```python
from build123d import *

# Parameters (mm, degrees)
SKETCH_1_W                         = 7.5
SKETCH_1_H                         = 4.2
EXTRUDE_1_DEPTH                    = 6
CUT_EXTRUDE_1_DEPTH                = 5
CUT_EXTRUDE_2_DEPTH                = 11.482843126
EXTRUDE_6_DEPTH                    = 1.1
CUT_EXTRUDE_3_REACH                = 12.483
SKETCH_5_W                         = 5.3
SKETCH_5_H                         = 4.3
EXTRUDE_3_REACH                    = 12.131
EXTRUDE_5_REACH                    = 13.88
SKETCH_11_W                        = 2
SKETCH_11_H                        = 4.2
SKETCH_11_W_2                      = 0.8
SKETCH_11_H_2                      = 0.8
CUT_EXTRUDE_5_DEPTH                = 0.1
SKETCH_15_R                        = 0.05
CUT_EXTRUDE_6_DEPTH                = 0.1
CUT_EXTRUDE_7_DEPTH                = 0.2
SKETCH_7_W                         = 0.6
SKETCH_7_H                         = 0.6
EXTRUDE_4_DEPTH                    = 5.5
SKETCH_18_W                        = 0.6
SKETCH_18_H                        = 0.6
CHAMFER_6_SIZE                     = 0.2
PATTERN_LINEAR_1_COUNT             = 2
PATTERN_LINEAR_1_PITCH             = 2.5
CHAMFER_6_OF_PATTERN_LINEAR_1_SIZE = 0.2
CUT_EXTRUDE_4_REACH                = 12.131
SKETCH_20_W                        = 0.6
SKETCH_20_H                        = 0.3
CUT_EXTRUDE_9_DEPTH                = 0.9
CHAMFER_5_SIZE                     = 0.3
SKETCH_19_R                        = 0.05
CUT_EXTRUDE_8_DEPTH                = 3.2


with BuildPart() as part:
    # Эскиз1 → Бобышка-Вытянуть1 (new body)
    with BuildSketch(Plane(origin=(0, 0, 0), x_dir=(1, 0, 0), z_dir=(0, 1, 0))):
        with Locations((3.75, -2.1)):
            Rectangle(SKETCH_1_W, SKETCH_1_H)
    extrude(amount=EXTRUDE_1_DEPTH)

    # Эскиз2 → Вырез-Вытянуть1 (cut)
    with BuildSketch(Plane(origin=(0, 6, 0), x_dir=(1, 0, 0), z_dir=(0, 1, 0))):
        Polygon((0.5, -0.9), (7, -0.9), (7, -1.9), (6.4, -1.9), (6.4, -3.7), (1.1, -3.7), (1.1, -1.9), (0.5, -1.9), align=None)
    extrude(amount=-CUT_EXTRUDE_1_DEPTH, mode=Mode.SUBTRACT)

    # Эскиз3 → Вырез-Вытянуть2 (cut, through all)
    with BuildSketch(Plane.ZY):
        Polygon((2.2, 6), (2.2, 1.5), (2.7, 1.5), (3.1, 3.459591794), (3.1, 4.021282026), (2.8, 4.285857157), (2.8, 4.585857157), (3.5, 5.3), (4.2, 5.3), (4.2, 6), align=None)
    extrude(amount=-CUT_EXTRUDE_2_DEPTH, mode=Mode.SUBTRACT)

    # Эскиз16 → Бобышка-Вытянуть6 (add)
    with BuildSketch(Plane(origin=(7.5, 0, 0), x_dir=(0, 0, -1), z_dir=(1, 0, 0))):
        Polygon((-2.4, 0), (-1.3, -2.2), (0, -2.2), (0, 0), align=None)
    extrude_6 = extrude(amount=-EXTRUDE_6_DEPTH)

    # Зеркальное отражение2: Бобышка-Вытянуть6 across plane
    add(extrude_6.mirror(Plane(origin=(3.75, 0, 0), x_dir=(0, 0, 1), z_dir=(1, 0, 0))))

    # Эскиз5 → Вырез-Вытянуть3 (cut, up to next)
    with BuildSketch(Plane.XY.offset(4.2), mode=Mode.PRIVATE) as cut_extrude_3_sk1:
        with Locations((3.75, 3.15)):
            Rectangle(SKETCH_5_W, SKETCH_5_H)
    cut_extrude_3_tool1 = extrude(cut_extrude_3_sk1.sketch, amount=-CUT_EXTRUDE_3_REACH, mode=Mode.PRIVATE) & part.part
    add(cut_extrude_3_tool1.solids().sort_by_distance((3.75, 3.15, 4.2))[0], mode=Mode.SUBTRACT)

    # Эскиз6 → Бобышка-Вытянуть3 (add, up to next)
    with BuildSketch(Plane(origin=(0.5, 0, 0), x_dir=(0, 0, -1), z_dir=(1, 0, 0)), mode=Mode.PRIVATE) as extrude_3_sk1:
        Polygon((-3.3, 1), (-2.67, 1.5), (-0.9, 1.5), (-0.9, 1), align=None)
    extrude_3_tool1 = extrude(extrude_3_sk1.sketch, amount=EXTRUDE_3_REACH, mode=Mode.PRIVATE) - part.part
    add(extrude_3_tool1.solids().sort_by_distance((0.5, 1.23741, 1.950432))[0])

    # Эскиз9 → Бобышка-Вытянуть5 (add, up to next)
    with BuildSketch(Plane(origin=(0, 6, 0), x_dir=(1, 0, 0), z_dir=(0, 1, 0)), mode=Mode.PRIVATE) as extrude_5_sk1:
        Polygon((3.45, -0.9), (3.75, -1.328444402), (4.05, -0.9), align=None)
    extrude_5_tool1 = extrude(extrude_5_sk1.sketch, amount=-EXTRUDE_5_REACH, mode=Mode.PRIVATE) - part.part
    add(extrude_5_tool1.solids().sort_by_distance((3.75, 6, 1.042815))[0])

    # Эскиз11 → Вырез-Вытянуть5 (cut)
    with BuildSketch(Plane.XZ):
        with Locations((2.5, 2.1)):
            Rectangle(SKETCH_11_W, SKETCH_11_H)
        with Locations((2.5, 2)):
            Rectangle(SKETCH_11_W_2, SKETCH_11_H_2, mode=Mode.SUBTRACT)
    cut_extrude_5 = extrude(amount=-CUT_EXTRUDE_5_DEPTH, mode=Mode.SUBTRACT)

    # Эскиз15 → Вырез-Вытянуть6 (cut)
    with BuildSketch(Plane.XZ):
        with Locations(Location((2.5, 2, 0), (0, 0, 270))):
            Circle(SKETCH_15_R)
    extrude(amount=-CUT_EXTRUDE_6_DEPTH, mode=Mode.SUBTRACT)

    # Эскиз17 → Вырез-Вытянуть7 (cut)
    with BuildSketch(Plane.XY.offset(4.2)):
        Polygon((0.55, 5), (0.15, 4.307179677), (0.95, 4.307179677), align=None)
    extrude(amount=-CUT_EXTRUDE_7_DEPTH, mode=Mode.SUBTRACT)

    # Эскиз7 → Бобышка-Вытянуть4 (add)
    with BuildSketch(Plane.XZ):
        with Locations((2.5, 2)):
            Rectangle(SKETCH_7_W, SKETCH_7_H)
    extrude_4 = extrude(amount=-EXTRUDE_4_DEPTH)

    # По траектории1: sweep along a curve in space
    with BuildLine() as sweep_1_path:
        Line((2.5, -0.7, 1.3), (2.5, -0.7, -3.2))
        ThreePointArc((2.5, 0, 2), (2.5, -0.494974747, 1.794974747), (2.5, -0.7, 1.3))
    # Эскиз18 → По траектории1 (sweep)
    with BuildSketch(Plane.XZ):
        with Locations((2.5, 2)):
            Rectangle(SKETCH_18_W, SKETCH_18_H)
    sweep_1 = sweep(path=sweep_1_path.line)

    # Фаска6
    chamfer_6_edges = [part.edges().sort_by_distance(p)[0] for p in [
        (2.8, 5.5, 2),
        (2.5, 5.5, 1.7),
        (2.2, 5.5, 2),
        (2.5, 5.5, 2.3),
        (2.8, -0.7, -3.2),
        (2.5, -1, -3.2),
        (2.2, -0.7, -3.2),
        (2.5, -0.4, -3.2),
    ]]
    chamfer(chamfer_6_edges, length=CHAMFER_6_SIZE)

    # Линейный массив1: Вырез-Вытянуть5, Бобышка-Вытянуть4, По траектории1 ×2
    with Locations(*[(i * PATTERN_LINEAR_1_PITCH, 0, 0) for i in range(1, PATTERN_LINEAR_1_COUNT)]):
        add(cut_extrude_5, mode=Mode.SUBTRACT)
        add(extrude_4)
        add(sweep_1)

    # Фаска6 of Линейный массив1
    chamfer_6_of_pattern_linear_1_edges = [part.edges().sort_by_distance(p)[0] for p in [
        (5.3, 5.5, 2),
        (5, 5.5, 1.7),
        (4.7, 5.5, 2),
        (5, 5.5, 2.3),
        (5.3, -0.7, -3.2),
        (5, -1, -3.2),
        (4.7, -0.7, -3.2),
        (5, -0.4, -3.2),
    ]]
    chamfer(chamfer_6_of_pattern_linear_1_edges, length=CHAMFER_6_OF_PATTERN_LINEAR_1_SIZE)

    # Вырез-Вытянуть4: up to this plane
    cut_extrude_4_end = Plane(origin=(4.05, -2.202, 0.9), z_dir=(0.8191520442889916, 0, 0.5735764363510465))
    # Эскиз10 → Вырез-Вытянуть4 (cut, up to the surface)
    with BuildSketch(Plane(origin=(0.5, 0, 0), x_dir=(0, 0, -1), z_dir=(1, 0, 0)), mode=Mode.PRIVATE) as cut_extrude_4_sk1:
        Polygon((-1.4, 6), (-0.9, 6), (-1.4, 5.5), align=None)
    cut_extrude_4_tool1 = split(extrude(cut_extrude_4_sk1.sketch, amount=CUT_EXTRUDE_4_REACH, mode=Mode.PRIVATE), bisect_by=cut_extrude_4_end, keep=Keep.BOTH, mode=Mode.PRIVATE)
    add(cut_extrude_4_tool1.solids().sort_by_distance((0.5, 5.833333, 1.233333))[0], mode=Mode.SUBTRACT)

    # Эскиз20 → Вырез-Вытянуть9 (cut)
    with BuildSketch(Plane(origin=(0, 6, 0), x_dir=(1, 0, 0), z_dir=(0, 1, 0))):
        with Locations((0.8, -2.05)):
            Rectangle(SKETCH_20_W, SKETCH_20_H)
    cut_extrude_9 = extrude(amount=-CUT_EXTRUDE_9_DEPTH, mode=Mode.SUBTRACT)

    # Зеркальное отражение3: Вырез-Вытянуть9 across plane
    add(cut_extrude_9.mirror(Plane(origin=(3.75, 0, 0), x_dir=(0, 0, 1), z_dir=(1, 0, 0))), mode=Mode.SUBTRACT)

    # Фаска5
    chamfer_5_edges = [part.edges().sort_by_distance(p)[0] for p in [
        (0.5, 6, 1.55),
        (7, 6, 1.55),
    ]]
    chamfer(chamfer_5_edges, length=CHAMFER_5_SIZE)

    # Эскиз19 → Вырез-Вытянуть8 (cut)
    with BuildSketch(Plane(origin=(0, 0, 0), x_dir=(-1, 0, 0), z_dir=(0, 0, -1))):
        with Locations(Location((-2.5, -0.7, 0), (0, 0, 270))):
            Circle(SKETCH_19_R)
    extrude(amount=CUT_EXTRUDE_8_DEPTH, mode=Mode.SUBTRACT)


solid = part.part
```
Here's how the part is built. I have some questions about the finished solid (model axes, mm). A direction names the side the tool comes from. Coordinates: 2 decimals unless noted, no trailing zeros. Write each loop counter-clockwise with the first axis right and the second up, starting at its lowest first coordinate (ties: lowest second). Pieces come first, ordered by that corner, then holes. Notation, with made-up numbers: (45.25, 20.25) -> (73.25, 20.25) arc R10 ccw to (73.25, 29.25) -> close; hole circle Ø8 at (9, -12). An arc over 180 degrees is marked (long way). Use a Markdown table: item, result. Add a question column.
(1) Please list where these lines run through material, in increasing order: line 1 (Z direction, x = 5, y = 1.75); line 2 (X direction, y = -0.5, z = -1); line 3 (Z direction, x = 2, y = 5).
(2) For faces 4 (the flat face through (5, 0.1, 3)), 5 (the cylindrical face through (4.996, -0.699, 2.015)), 6 (the flat face through (7, 3, 2.2)), 7 (the flat face through (6.4, -1, 1)), which set-ups out of +Z, -Z, +X, -X, +Y, -Y let a thin tool reach every point of the face, with its end or its side?
(3) If we section it at B-B, the plane y = 3.25: State how many separate pieces and enclosed holes the cut face has, and give its area (3 significant figures).
(4) If we section it at A-A, the plane z = -0.5: Write out the boundary of the cut face in (x, y), and give its area (3 significant figures).
(5) We'd pull the mould along Z, two halves only. Please class faces 1 (the flat face through (2, 4, 0.9)), 2 (the flat face through (4, 3, 0)), 3 (the flat face through (1.1, -1, 1)): +Z half, -Z half, draft (parallel to the pull), parting line (faces both ways), or undercut.
(6) I'm going to push flat-ended pins straight in: P1, Ø2, axis at x = 6, z = -1, coming from the -Y side; P2, Ø1.1, axis at y = -0.5, z = -1.5, coming from the -X side; P3, Ø3, axis at x = 1, y = 4, coming from the -Z side; P4, Ø3, axis at y = 0.5, z = -1, coming from the -X side. Where does each tip first touch, or does it pass through?
(7) If we section it at C-C, the plane y = 1.25: Write out the boundary of the cut face in (x, z) (3 decimals).
Outcome:
| question | item | result |
|---|---|---|
| 1 | line 1 | z = 0 to 0.9, 1.7 to 2.3 |
| 1 | line 2 | x = 2.2 to 2.8, 4.7 to 5.3 |
| 1 | line 3 | z = 0 to 0.9 |
| 2 | face 4 | none |
| 2 | face 5 | +Z, -Y |
| 2 | face 6 | +X, +Y |
| 2 | face 7 | +Z, -Z, -Y |
| 3 | separate pieces | 5 |
| 3 | enclosed holes | 0 |
| 3 | area | 11.8 mm^2 |
| 4 | outline | (2.2, -1) -> (2.8, -1) -> (2.8, -0.4) -> (2.2, -0.4) -> close; (4.7, -1) -> (5.3, -1) -> (5.3, -0.4) -> (4.7, -0.4) -> close; hole circle Ø0.1 at (2.5, -0.7) |
| 4 | area | 0.712 mm^2 |
| 5 | face 1 | undercut |
| 5 | face 2 | -Z half |
| 5 | face 3 | draft |
| 6 | P1 | stops at y = -1 |
| 6 | P2 | stops at x = 2.2 |
| 6 | P3 | stops at z = 0 |
| 6 | P4 | stops at x = 0 |
| 7 | outline | (0, 0) -> (7.5, 0) -> (7.5, 4.2) -> (6.4, 4.2) -> (6.4, 2.985) -> (1.1, 2.985) -> (1.1, 4.2) -> (0, 4.2) -> close |
